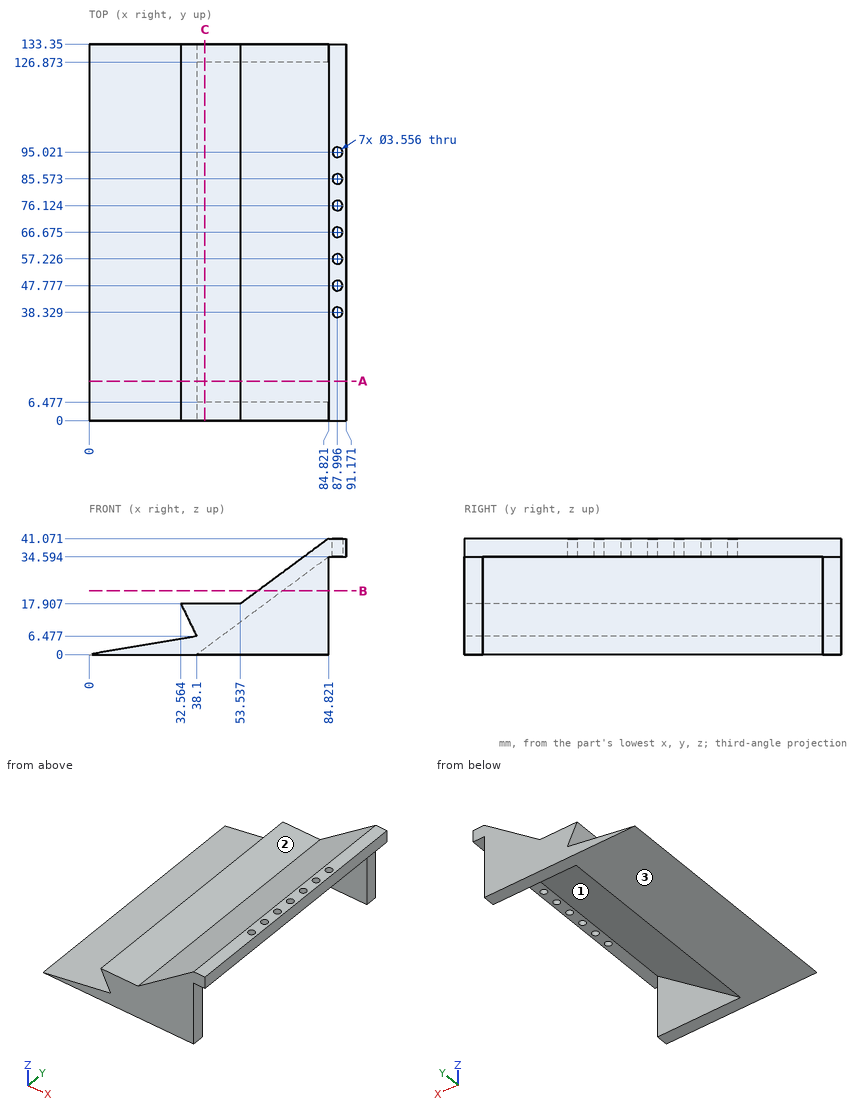
Geometry: see drawing. Coordinates: mm, zero at the bounding-box minimum. A direction names the side the tool comes from. Coordinates: 2 decimals unless noted, no trailing zeros. Order: outer loops, then holes, each group sorted by start corner. A loop starts at its lowest first (then second) coordinate and runs counter-clockwise, first axis right, second up. Notation, with made-up numbers: (19, -1.5) - (61, -1.5) arc R21 ccw to (61, 36.5) - close; hole circle Ø8 at (-28, -18). An arc over 180 degrees is marked (long way). Return JSON: item names as keys, results as strings.
Q1. Cut plane C-C (x = 41). Return loops of the section in (y, z), then the cut area to 3 significant figures.
The answers:
{"outline": "(0, 0) - (6.48, 0) - (6.48, 2.15) - (126.87, 2.15) - (126.87, 0) - (133.35, 0) - (133.35, 17.91) - (0, 17.91) - close", "area": "2,130 mm2"}
Q2. First-contact query: pin 1 (4 mm diameter, centred on x = 88, y = 38.33, fed in from -Z); pin 2 (17 mm diameter, centred on x = 40.5, y = 85.5, fed in from +Z); pin 3 (1 mm diameter, centred on x = 69.5, y = 47.5, fed in from -Z); pin 4 (2 mm diameter, centred on x = 88, y = 57.23, fed in from +Z). Flat tips, straight axial feed; report the tip coordinate or a pass-through.
The answers:
{"pin 1": "stops at z = 34.59", "pin 2": "stops at z = 17.91", "pin 3": "stops at z = 22.88", "pin 4": "passes through"}
Q3. Cut plane A-A (y = 14). Return loops of the section in (x, z) (1 decimal).
The answers:
{"outline": "(0, 0) - (38.1, 0) - (84.8, 34.6) - (91.2, 34.6) - (91.2, 41.1) - (84.8, 41.1) - (53.5, 17.9) - (32.6, 17.9) - (38.1, 6.5) - close"}
Q4. Access query for the marked faces 1, 2 and 3. Directions: +Z, -Z, +X, -X, +Y, -Y. A direction counts if a zero-diameter tool reaches every point of the face in a straight line with its end or side. Return the directions, or none.
The answers:
{"face 1": "-Z, +X", "face 2": "+Z, -X, +Y, -Y", "face 3": "-Z, +X, -X, +Y, -Y"}
Q5. Ray query, probe 1 along Y at (x, z) = (84.5, 14); probe 2 along Z at (x, y) = (86, 100.5); probe 3 along X at (y, z) = (32.5, 32) (1 decimal). Return the intervals inside material, ascending.
The answers:
{"probe 1": "y = 0 to 6.48, 126.87 to 133.35", "probe 2": "z = 34.59 to 41.07", "probe 3": "x = 72.6 to 81.3"}
Q6. Cut plane B-B (z = 22.5). Return loops of the section in (x, y), then the cut area to 3 significant figures.
The answers:
{"outline": "(59.74, 0) - (84.82, 0) - (84.82, 6.48) - (68.49, 6.48) - (68.49, 126.87) - (84.82, 126.87) - (84.82, 133.35) - (59.74, 133.35) - close", "area": "1,380 mm2"}
